Input: part model. Units: mm. Frame: model coordinates. A direction names the side the tool comes from. Give positions to 0.01 mm unless a question says otherwise; leave off trailing zeros. Write each loop counter-clockwise with the first axis right and the second up, starting at its lowest first coordinate (ties: lowest second). Pieces come first, ordered by that corner, then holes. Notation, with made-up numbers: (82, -38.75) - (87, -38.75) arc R20 cw to (87, -1.75) - close; hole circle Ø9 at (20.5, 30.5). An arc over 180 degrees is marked (long way). Answer as CSV lines item,"result".
```python
from build123d import *

# Parameters (mm, degrees)
SKETCH012_W   = 150
SKETCH012_H   = 120
SKETCH012_R   = 19.9
PAD004_DEPTH  = 2
SKETCH013_R   = 19.9
SKETCH013_R_2 = 17.9
PAD005_DEPTH  = 5
SKETCH014_R   = 54.1
SKETCH014_R_2 = 50.1
PAD006_DEPTH  = 5


with BuildPart() as part:
    # Sketch012 → Pad004 (new body)
    with BuildSketch(Plane.YZ):
        Rectangle(SKETCH012_W, SKETCH012_H)
        Circle(SKETCH012_R, mode=Mode.SUBTRACT)
    extrude(amount=PAD004_DEPTH)

    # Sketch013 → Pad005 (join)
    with BuildSketch(Plane.YZ):
        Circle(SKETCH013_R)
        Circle(SKETCH013_R_2, mode=Mode.SUBTRACT)
    extrude(amount=PAD005_DEPTH)

    # Sketch014 → Pad006 (join)
    with BuildSketch(Plane.YZ):
        Circle(SKETCH014_R)
        Circle(SKETCH014_R_2, mode=Mode.SUBTRACT)
    extrude(amount=PAD006_DEPTH)


solid = part.part
```
Item 1: Reachability of faces 1 (the face through (0, -18, -12)), 2 (the face through (2, -18, 54)) from +Z, -Z, +X, -X, +Y, -Y: full face, straight path, thin tool, end or side. Return the list, or none.
The answers:
face 1,"+Z, -Z, -X, +Y, -Y"
face 2,"+X"
Item 2: Cut plane B-B on y = 0. Return the cut outline in (x, z).
The answers:
outline,"(0, -60) - (2, -60) - (2, -54.1) - (5, -54.1) - (5, -50.1) - (2, -50.1) - (2, -19.9) - (5, -19.9) - (5, -17.9) - (0, -17.9) - close; (0, 17.9) - (5, 17.9) - (5, 19.9) - (2, 19.9) - (2, 50.1) - (5, 50.1) - (5, 54.1) - (2, 54.1) - (2, 60) - (0, 60) - close"
Item 3: Cut plane C-C on x = 3.15. Return the cut outline in (y, z).
The answers:
outline,"circle Ø108.2 at (0, 0); circle Ø39.8 at (0, 0); hole circle Ø100.2 at (0, 0); hole circle Ø35.8 at (0, 0)"
Item 4: Cut plane A-A on z = 0. Return the cut outline in (x, y).
The answers:
outline,"(0, -75) - (2, -75) - (2, -54.1) - (5, -54.1) - (5, -50.1) - (2, -50.1) - (2, -19.9) - (5, -19.9) - (5, -17.9) - (0, -17.9) - close; (0, 17.9) - (5, 17.9) - (5, 19.9) - (2, 19.9) - (2, 50.1) - (5, 50.1) - (5, 54.1) - (2, 54.1) - (2, 75) - (0, 75) - close"
Item 5: Mould query, pull axis Y, two halves, no side actions, for faces 3 (the face through (2, -1, -22)), 4 (the face through (5, -18, 3)), 5 (the face through (3.48, -42.93, -32.92)). Classes: +Y half, -Y half, draft (parallel to the pull), parting line (faces both ways), or undercut.
The answers:
face 3,"undercut"
face 4,"draft"
face 5,"parting line"
Item 6: Cut plane D-D on y = -36.5. Return the cut outline in (x, z), plus the area to 3 significant figures.
The answers:
outline,"(0, -60) - (2, -60) - (2, -39.93) - (5, -39.93) - (5, -34.32) - (2, -34.32) - (2, 34.32) - (5, 34.32) - (5, 39.93) - (2, 39.93) - (2, 60) - (0, 60) - close"
area,"274 mm²"
Item 7: Ray query, line 1 (Z direction, x = 3.35, y = 0); line 2 (Y direction, x = 4.6, z = -5); line 3 (Y direction, x = 3.4, z = 2.5). Return the intervals inside material, ascending. Write a range as from..to.
The answers:
line 1,"-54.1..-50.1, -19.9..-17.9, 17.9..19.9, 50.1..54.1"
line 2,"-53.87..-49.85, -19.26..-17.19, 17.19..19.26, 49.85..53.87"
line 3,"-54.04..-50.04, -19.74..-17.72, 17.72..19.74, 50.04..54.04"
Item 8: Contact query for flat-ended pins moving along their axis: pin 1 (10 mm diameter, centred on y = 29, z = 32, fed in from +X); pin 2 (1.5 mm diameter, centred on x = 4, y = -42.5, fed in from +Z). Output: stop coordinate, or through.
The answers:
pin 1,"x = 2"
pin 2,"z = 34.41"
